```python
from build123d import *

# Parameters (mm, degrees)
SKETCH2_W               = 88.9
SKETCH2_H               = 152.4
BOSS_EXTRUDE1_DEPTH     = 5.9944
CUT_EXTRUDE2_DEPTH      = 177.535840076
CUT_EXTRUDE2_DEPTH_BACK = 177.535840076
SKETCH4_R               = 2.7305
BOSS_EXTRUDE2_DEPTH     = 101.6
FILLET1_R               = 3.81
FILLET2_R               = 2.54
BOSS_EXTRUDE3_DEPTH     = 20.32
FILLET3_R               = 3.81
FILLET6_R               = 3.81
FILLET7_R               = 2.54
CUT_EXTRUDE3_DEPTH      = 204.596488182
CUT_EXTRUDE3_DEPTH_BACK = 204.596488182
SKETCH7_W               = 2.54
SKETCH7_H               = 152.4
SKETCH8_W               = 86.36
SKETCH8_H               = 152.4
CUT_EXTRUDE5_DEPTH      = 5.9944
SKETCH9_R               = 0.79375
CUT_EXTRUDE6_DEPTH      = 3.175


with BuildPart() as part:
    # Sketch2 → Boss-Extrude1 (new body)
    with BuildSketch(Plane(origin=(0, 0, 0), x_dir=(1, 0, 0), z_dir=(0, 1, 0))):
        with Locations((44.45, 76.2)):
            Rectangle(SKETCH2_W, SKETCH2_H)
    extrude(amount=BOSS_EXTRUDE1_DEPTH)

    # Sketch4 → Cut-Extrude2 (cut, two sides: drawn at the far end of the back side and taken through both)
    with BuildSketch(Plane(origin=(0, 5.9944, 0), x_dir=(1, 0, 0), z_dir=(0, 1, 0)).offset(-CUT_EXTRUDE2_DEPTH_BACK)):
        with Locations(Location((45.72, 109.871331367, 0), (0, 0, 270))):
            Circle(SKETCH4_R)
        with Locations(Location((45.72, 33.671331367, 0), (0, 0, 270))):
            Circle(SKETCH4_R)
    extrude(amount=CUT_EXTRUDE2_DEPTH + CUT_EXTRUDE2_DEPTH_BACK, mode=Mode.SUBTRACT)

    # Sketch5 → Boss-Extrude2 (add)
    with BuildSketch(Plane(origin=(0, 5.9944, 0), x_dir=(1, 0, 0), z_dir=(0, 1, 0))):
        Polygon((18.542, 15.748), (12.446, 15.748), (12.446, 2.54), (76.454, 2.54), (76.454, 15.748), (70.358, 15.748), (70.358, 13.208), (71.374, 13.208), (71.374, 11.43), (70.358, 11.43), (70.358, 7.62), (18.542, 7.62), (18.542, 11.43), (17.526, 11.43), (17.526, 13.208), (18.542, 13.208), align=None)
    extrude(amount=BOSS_EXTRUDE2_DEPTH)

    # Fillet1
    fillet1_edges = [part.edges().sort_by_distance(p)[0] for p in [
        (12.446, 56.7944, -15.748),
        (12.446, 56.7944, -2.54),
        (76.454, 56.7944, -2.54),
        (76.454, 56.7944, -15.748),
    ]]
    fillet(fillet1_edges, radius=FILLET1_R)

    # Fillet2
    fillet2_edges = [part.edges().sort_by_distance(p)[0] for p in [
        (71.501, 5.9944, -15.748),
        (44.45, 5.9944, -2.54),
        (12.446, 5.9944, -9.144),
        (17.399, 5.9944, -15.748),
        (76.454, 5.9944, -9.144),
        (13.561923164, 5.9944, -3.655923164),
        (13.561923164, 5.9944, -14.632076836),
        (75.338076836, 5.9944, -3.655923164),
        (75.338076836, 5.9944, -14.632076836),
    ]]
    fillet(fillet2_edges, radius=FILLET2_R - 0.0001)  # a hair under: the kernel refuses the full size

    # Sketch6 → Boss-Extrude3 (add, symmetric)
    with BuildSketch(Plane.ZY.offset(-44.45)):
        Polygon((-149.86, 5.9944), (-79.121, 5.9944), (-79.121, 23.1394), (-86.106, 23.1394), (-86.106, 18.0594), (-84.201, 18.0594), (-84.201, 16.1544), (-86.106, 16.1544), (-86.106, 11.0744), (-142.875, 11.0744), (-142.875, 16.1544), (-144.78, 16.1544), (-144.78, 18.0594), (-142.875, 18.0594), (-142.875, 23.1394), (-149.86, 23.1394), align=None)
    extrude(amount=BOSS_EXTRUDE3_DEPTH, both=True)

    # Fillet3
    fillet3_edges = [part.edges().sort_by_distance(p)[0] for p in [
        (44.45, 23.1394, -149.86),
        (44.45, 23.1394, -79.121),
    ]]
    fillet(fillet3_edges, radius=FILLET3_R)

    # Fillet6
    fillet6_edges = [part.edges().sort_by_distance(p)[0] for p in [
        (24.13, 12.6619, -149.86),
        (64.77, 12.6619, -79.121),
        (24.13, 23.1394, -84.5185),
        (24.13, 12.6619, -79.121),
        (64.77, 23.1394, -84.5185),
        (64.77, 12.6619, -149.86),
        (64.77, 23.1394, -144.4625),
        (64.77, 22.023476836, -148.744076836),
        (64.77, 22.023476836, -80.236923164),
        (24.13, 23.1394, -144.4625),
        (24.13, 22.023476836, -148.744076836),
        (24.13, 22.023476836, -80.236923164),
    ]]
    fillet(fillet6_edges, radius=FILLET6_R)

    # Fillet7
    fillet7_edges = [part.edges().sort_by_distance(p)[0] for p in [
        (24.13, 5.9944, -114.4905),
        (64.77, 5.9944, -114.4905),
        (44.45, 5.9944, -79.121),
        (44.45, 5.9944, -149.86),
        (25.245923164, 5.9944, -80.236923164),
        (63.654076836, 5.9944, -80.236923164),
        (63.654076836, 5.9944, -148.744076836),
        (25.245923164, 5.9944, -148.744076836),
    ]]
    fillet(fillet7_edges, radius=FILLET7_R - 0.0001)  # a hair under: the kernel refuses the full size

    # Sketch7 → Cut-Extrude3 (cut, two sides: drawn at the far end of the back side and taken through both)
    with BuildSketch(Plane(origin=(0, 5.9944, 0), x_dir=(1, 0, 0), z_dir=(0, 1, 0)).offset(-CUT_EXTRUDE3_DEPTH_BACK)):
        with Locations((1.27, 76.2)):
            Rectangle(SKETCH7_W, SKETCH7_H)
    extrude(amount=CUT_EXTRUDE3_DEPTH + CUT_EXTRUDE3_DEPTH_BACK, mode=Mode.SUBTRACT)

    # Sketch8 → Cut-Extrude5 (cut)
    with BuildSketch(Plane.XZ):
        with Locations((45.72, -76.2)):
            Rectangle(SKETCH8_W, SKETCH8_H)
    extrude(amount=-CUT_EXTRUDE5_DEPTH, mode=Mode.SUBTRACT)


with BuildPart() as body_2:
    # of the pieces the cut leaves, the one that is kept (cut_extrude5_keep)
    add(part.part.solids().sort_by_distance((18.542, 8.5343, -15.748))[0])

    # Sketch9 → Cut-Extrude6 (cut)
    with BuildSketch(Plane.XZ.offset(-5.9944)):
        with Locations(Location((69.85, -5.08, 0), (0, 0, 270))):
            Circle(SKETCH9_R)
        with Locations(Location((19.05, -5.08, 0), (0, 0, 270))):
            Circle(SKETCH9_R)
    extrude(amount=-CUT_EXTRUDE6_DEPTH, mode=Mode.SUBTRACT)


solid = body_2.part
```
The listing builds one solid part. Answer for the finished solid, in the listing's coordinates (mm). A direction names the side the tool comes from. Round coordinates to 2 decimals unless told otherwise and drop trailing zeros. Loops run counter-clockwise (first coordinate to the right, second up) from the corner with the lowest first, then second, coordinate; pieces in that order, holes last.
Q1. Which of the six approach directions +Z, -Z, +X, -X, +Y, -Y give full straight-line access (tool end or side, diameter ignored) to faces 4 (the face through (12.446, 57, -9)), 5 (the face through (75.37, 58.76, -14.6)), 6 (the face through (18.542, 56, -15)), 7 (the face through (13.53, 58.76, -3.69)), 8 (the face through (72, 57, -15.748))?
Q2. Section A-A, the plane x = 34 is taken. Determine the outline of the cut face in (y, z), then the cut area to 3 significant figures.
Q3. Find the intervals of material crossed by line 1 (X direction, y = 8.05, z = -5.08); line 2 (Z direction, x = 70.5, y = 77.5); line 3 (X direction, y = 7.1, z = -5.08), in increasing order.
Q4. Given pin 1 Ø0.9 at (y, z) = (49.5, -12.5) entering from +X; pin 2 Ø1.4 at (y, z) = (66.5, -12) entering from -X; pin 3 Ø1.1 at (x, y) = (18, 46) entering from -Z, each flat-ended and moving along its own axis, determine where each tip first touches the part or whether it passes through.
Q5. For a pull along X with two mould halves and no side action, classify faces 1 (the face through (11.682, 6.719, -9.105)), 2 (the face through (70.358, 56, -10)), 3 (the face through (44.84, 6.72, -1.78)) as released by +X, released by -X, zero draft, split by the parting line, or undercut.
Q6. Section B-B, the plane y = 43 is taken. Determine the outline of the cut face in (x, z).
Completed:
1. face 4: +Z, -Z, -X, +Y
1. face 5: -Z, +X, +Y
1. face 6: -Z, +Y, -Y
1. face 7: +Z, -X, +Y
1. face 8: -Z, +X, -X, +Y
2. outline: (5.99, -7.62) - (107.59, -7.62) - (107.59, -2.54) - (8.53, -2.54) arc R2.54 cw to (5.99, 0) - close
2. area: 518 mm2
3. line 1: x = 12.61 to 18.26, 19.84 to 69.06, 70.64 to 76.29
3. line 2: z = -15.75 to -13.21, -11.43 to -2.54
3. line 3: x = 12.2 to 18.26, 19.84 to 69.06, 70.64 to 76.7
4. pin 1: stops at x = 76.45
4. pin 2: stops at x = 12.45
4. pin 3: stops at z = -15.75
5. face 1: released by -X
5. face 2: undercut
5. face 3: zero draft
6. outline: (12.45, -11.94) arc R3.81 ccw to (16.26, -15.75) - (18.54, -15.75) - (18.54, -13.21) - (17.53, -13.21) - (17.53, -11.43) - (18.54, -11.43) - (18.54, -7.62) - (70.36, -7.62) - (70.36, -11.43) - (71.37, -11.43) - (71.37, -13.21) - (70.36, -13.21) - (70.36, -15.75) - (72.64, -15.75) arc R3.81 ccw to (76.45, -11.94) - (76.45, -6.35) arc R3.81 ccw to (72.64, -2.54) - (16.26, -2.54) arc R3.81 ccw to (12.45, -6.35) - close
